Study the drawing (mm; zero at the part's minimum x, y, z) and answer. A direction names the side the tool comes from. Coordinates: 2 decimals unless noted, no trailing zeros. Order: outer loops, then holes, each group sorted by start corner. A loop starts at its lowest first (then second) coordinate and runs counter-clockwise, first axis right, second up. Notation, with made-up numbers: (78.5, 72.25) -> (130.5, 72.25) arc R12 cw to (130.5, 93.25) -> close; hole circle Ø10 at (-30, -26). An arc over 180 degrees is marked (long way). Put each result on its own line as item: value. Start each with the question number.
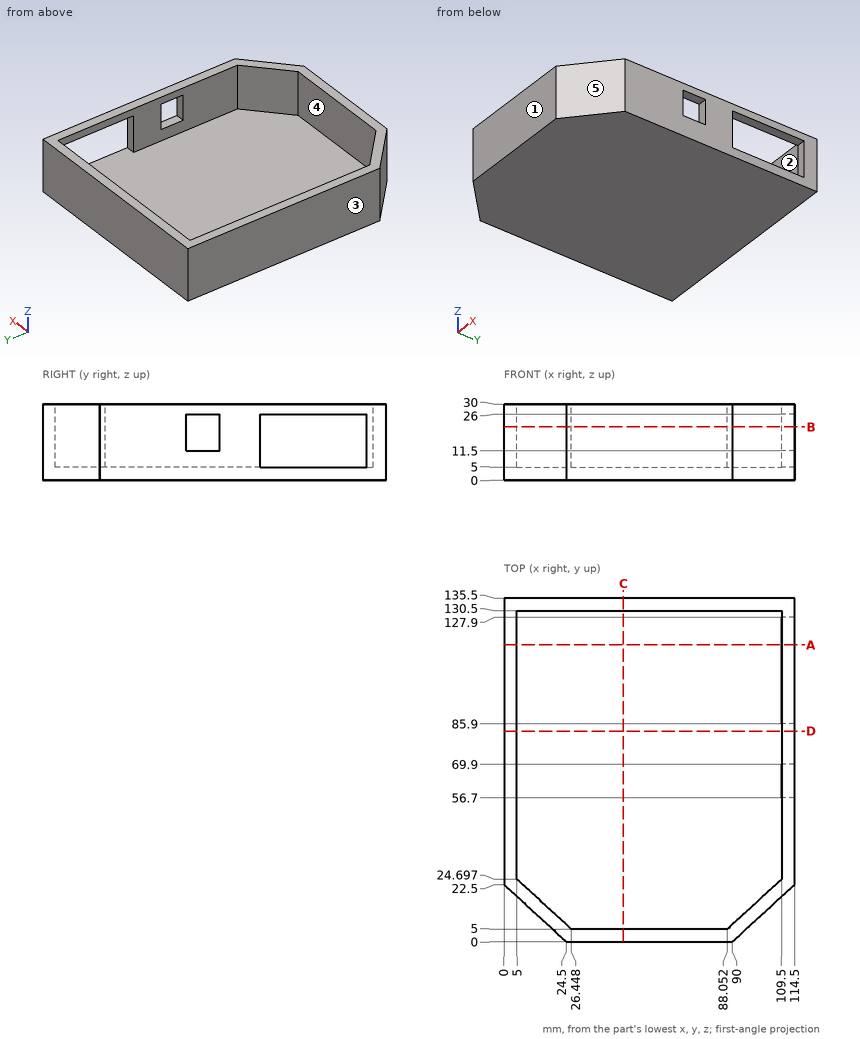
(1) Each of these flat-tipped pins is pushed along its axis until it touches: P1, Ø6, axis at x = 90, y = 81, coming from the +Z side; P2, Ø1.5, axis at x = 111, z = 10.5, coming from the -Y side; P3, Ø4, axis at x = 111, z = 22, coming from the -Y side. Where does it stop, or does it pass through?
(2) The part is cut by section A-A on y = 117. Determine the outline of the cut face in (x, z).
(3) The part is cut by section D-D on y = 83. Determine the outline of the cut face in (x, z).
(4) The part is cut by section C-C on x = 47. Determine the outline of the cut face in (y, z).
(5) For a pull along Y with two mould halves and no side action, classify the marked faces 3, 4 and 5 as released by +Y, released by -Y, zero draft, split by the parting line, or undercut.
(6) A tool of negligible diameter and unlimited length cuts with its end or side. For the marked faces 1 and 2, from which of +Z, -Z, +X, -X, +Y, -Y can it reach the whole face along a straight path? Write none if from no direction.
(7) Find the intervals of material crossed by L1, parallel to X at y = 128, z = 6.25; L2, parallel to Y at x = 37, z = 7.5; L3, parallel to Z at x = 37.5, y = 49, in increasing order.
(8) The part is cut by section B-B on z = 21. Determine the outline of the cut face in (x, y).
Worked out:
1. P1: z = 5
1. P2: y = 18.6
1. P3: y = 17.45
2. outline: (0, 0) -> (114.5, 0) -> (114.5, 5) -> (5, 5) -> (5, 30) -> (0, 30) -> close; (109.5, 26) -> (114.5, 26) -> (114.5, 30) -> (109.5, 30) -> close
3. outline: (0, 0) -> (114.5, 0) -> (114.5, 30) -> (109.5, 30) -> (109.5, 5) -> (5, 5) -> (5, 30) -> (0, 30) -> close
4. outline: (0, 0) -> (135.5, 0) -> (135.5, 30) -> (130.5, 30) -> (130.5, 5) -> (5, 5) -> (5, 30) -> (0, 30) -> close
5. face 3: zero draft
5. face 4: undercut
5. face 5: released by -Y
6. face 1: +Z, -Z, +X, -X, -Y
6. face 2: +Z
7. L1: 0 to 5, 109.5 to 114.5
7. L2: 0 to 5, 130.5 to 135.5
7. L3: 0 to 5
8. outline: (0, 22.5) -> (24.5, 0) -> (90, 0) -> (114.5, 22.5) -> (114.5, 56.7) -> (109.5, 56.7) -> (109.5, 24.7) -> (88.05, 5) -> (26.45, 5) -> (5, 24.7) -> (5, 130.5) -> (109.5, 130.5) -> (109.5, 127.9) -> (114.5, 127.9) -> (114.5, 135.5) -> (0, 135.5) -> close; (109.5, 69.9) -> (114.5, 69.9) -> (114.5, 85.9) -> (109.5, 85.9) -> close
